Design review of the part built by this model. Coordinates are the model's own, in mm. A direction names the side the tool comes from. Coordinates: 2 decimals unless noted, no trailing zeros. Write each loop counter-clockwise with the first axis right and the second up, starting at its lowest first coordinate (ties: lowest second). Pieces come first, ordered by that corner, then holes. Notation, with made-up numbers: (70, 82) -> (102, 82) arc R21 ccw to (102, 87) -> close; hole circle Ø8 at (78, -27). An arc over 180 degrees is marked (long way). Return JSON: item names as keys, results as strings. Group by question number.
from build123d import *

# Parameters (mm, degrees)
SALIENTE_EXTRUIR1_DEPTH    = 105
SALIENTE_EXTRUIR2_DEPTH    = 5
CROQUIS3_W                 = 140
CROQUIS3_H                 = 105
SALIENTE_EXTRUIR3_DEPTH    = 5
CROQUIS4_W                 = 205
CROQUIS4_H                 = 105
SALIENTE_EXTRUIR5_DEPTH    = 5
CROQUIS5_W                 = 205
CROQUIS5_H                 = 105
SALIENTE_EXTRUIR6_DEPTH    = 5
SALIENTE_EXTRUIR7_DEPTH    = 140
CORTAR_EXTRUIR1_DEPTH      = 273.167228172
CORTAR_EXTRUIR1_DEPTH_BACK = 273.167228172
CROQUIS9_W                 = 20
CROQUIS9_H                 = 17.5
CROQUIS9_W_2               = 50
SALIENTE_EXTRUIR8_DEPTH    = 2.5
CROQUIS10_W                = 20
CROQUIS10_H                = 17.5
CROQUIS10_W_2              = 50
SALIENTE_EXTRUIR9_DEPTH    = 2.5
CORTAR_EXTRUIR2_START      = -5
CORTAR_EXTRUIR2_DEPTH      = 140


with BuildPart() as part:
    # Croquis2 → Saliente-Extruir1 (new body)
    with BuildSketch(Plane(origin=(0, 0, 0), x_dir=(1, 0, 0), z_dir=(0, 1, 0))):
        with BuildLine():
            Line((120, 70), (60, 70))
            add(Edge.make_bspline(
                [(60, 70), (89.76394683, -0.562785514), (120, 50)],
                knots=[0, 0, 0, 1, 1, 1], degree=2))
            Line((120, 50), (200, 50))
            Line((200, 50), (200, 70))
            Line((200, 70), (120, 70))
        make_face()
    extrude(amount=SALIENTE_EXTRUIR1_DEPTH)

    # Croquis2_3 → Saliente-Extruir2 (add)
    with BuildSketch(Plane(origin=(0, 0, 0), x_dir=(1, 0, 0), z_dir=(0, 1, 0))):
        with BuildLine():
            Line((60, 70), (60, -70))
            Line((60, -70), (200, -70))
            Line((200, -70), (200, 50))
            Line((200, 50), (120, 50))
            add(Edge.make_bspline(
                [(60, 70), (89.76394683, -0.562785514), (120, 50)],
                knots=[0, 0, 0, 1, 1, 1], degree=2))
        make_face()
    extrude(amount=SALIENTE_EXTRUIR2_DEPTH)

    # Croquis3 → Saliente-Extruir3 (add)
    with BuildSketch(Plane(origin=(200, 0, 0), x_dir=(0, 0, -1), z_dir=(1, 0, 0))):
        with Locations((0, 52.5)):
            Rectangle(CROQUIS3_W, CROQUIS3_H)
    extrude(amount=SALIENTE_EXTRUIR3_DEPTH)

    # Croquis4 → Saliente-Extruir5 (add)
    with BuildSketch(Plane.XY.offset(70)):
        with Locations((102.5, 52.5)):
            Rectangle(CROQUIS4_W, CROQUIS4_H)
    extrude(amount=SALIENTE_EXTRUIR5_DEPTH)

    # Croquis5 → Saliente-Extruir6 (add)
    with BuildSketch(Plane(origin=(0, 0, -70), x_dir=(-1, 0, 0), z_dir=(0, 0, -1))):
        with Locations((-102.5, 52.5)):
            Rectangle(CROQUIS5_W, CROQUIS5_H)
    extrude(amount=SALIENTE_EXTRUIR6_DEPTH)

    # Croquis6 → Saliente-Extruir7 (add)
    with BuildSketch(Plane.XY.offset(-70)):
        Polygon((60, 5), (0, 75), (0, 70), (60, 0), align=None)
    extrude(amount=SALIENTE_EXTRUIR7_DEPTH)

    # Croquis8 → Cortar-Extruir1 (cut, two sides: drawn at the far end of the back side and taken through both)
    with BuildSketch(Plane.XY.offset(-70).offset(-CORTAR_EXTRUIR1_DEPTH_BACK)):
        Polygon((60, 0), (0, 70), (0, 0), align=None)
    extrude(amount=CORTAR_EXTRUIR1_DEPTH + CORTAR_EXTRUIR1_DEPTH_BACK, mode=Mode.SUBTRACT)

    # Croquis9 → Saliente-Extruir8 (add)
    with BuildSketch(Plane.XY.offset(75)):
        with Locations((10, 87.5)):
            Rectangle(CROQUIS9_W, CROQUIS9_H)
        with Locations((-25, 87.5)):
            Rectangle(CROQUIS9_W_2, CROQUIS9_H)
    extrude(amount=-SALIENTE_EXTRUIR8_DEPTH)

    # Croquis10 → Saliente-Extruir9 (add)
    with BuildSketch(Plane(origin=(0, 0, -75), x_dir=(-1, 0, 0), z_dir=(0, 0, -1))):
        with Locations((-10, 87.5)):
            Rectangle(CROQUIS10_W, CROQUIS10_H)
        with Locations((25, 87.5)):
            Rectangle(CROQUIS10_W_2, CROQUIS10_H)
    extrude(amount=-SALIENTE_EXTRUIR9_DEPTH)

    # Croquis11 → Cortar-Extruir2 (cut)
    with BuildSketch(Plane(origin=(0, 105, 0), x_dir=(1, 0, 0), z_dir=(0, 1, 0)).offset(CORTAR_EXTRUIR2_START)):
        with BuildLine():
            Line((65.571134008, 70), (195, 70))
            Line((195, 70), (195, 55))
            Line((195, 55), (117.1633318, 55))
            add(Edge.make_bspline(
                [(117.1633318, 55), (116.553479191, 53.981059511), (115.34399458, 51.951404655), (113.624065501, 49.181454683), (110.189825419, 44.210450859), (105.056898876, 38.454652942), (100.423455416, 35.264929664), (97.501660631, 34.185491141), (95.327997633, 33.847005409), (93.19350491, 33.972145162), (90.391223635, 34.735002625), (85.948013808, 37.366168652), (78.790008493, 44.736062985), (74.164523658, 52.513426841)],
                knots=[-0.028793704, -0.028793704, -0.028793704, -0.004727786, 0.019338133, 0.06746997, 0.163733644, 0.292085209, 0.388348883, 0.452524666, 0.516700448, 0.580876231, 0.677139905, 0.80549147, 0.998018818, 0.998018818, 0.998018818], degree=2))
            Line((74.164523658, 52.513426841), (65.571134008, 70))
        make_face()
    extrude(amount=-CORTAR_EXTRUIR2_DEPTH, mode=Mode.SUBTRACT)


solid = part.part
Q1. Wall thickness on L1, parallel to Z at x = 110, y = 38; L2, parallel to Z at x = 87.5, y = 38.5; L3, parallel to X at y = 52, z = -50.5: over which ranges is each line inside the solid? List them lowest first.
Q2. For P1, Ø0.8, axis at x = -15.5, z = 73.5, coming from the -Y side; P2, Ø12, axis at x = 80, z = -5.5, coming from the +Y side; P3, Ø4.5, axis at y = 75, z = -62.5, coming from the -X side, all flat-tipped, find the tip position at first contact; note any pin that passes through.
Q3. We need section D-D on y = 54.5. State how many separate pieces and enclosed holes the cut face has, plus the area to 3 significant figures.
Q4. We need section B-B on z = 15.5. Write out the cut boundary in (x, y).
Q5. For faces 1 (the flat face through (157, 51, -55)), 2 (the flat face through (129, 5, 15)), 3 (the flat face through (-25, 88, 72.5)), list the 3-axis set-ups (+Z, -Z, +X, -X, +Y, -Y) from which the entire face can be reached by the end or side of a thin tool; tool diameter is ignored.
Q6. We need section A-A on x = -29.5. Write out the cut boundary in (y, z), plus the area to 3 significant figures.
Q7. We need section C-C on x = 148.5. Write out the cut boundary in (y, z), plus the area to 3 significant figures.
Q8. The part is to be moulded in two halves that separate along Z. For faces 4 (the flat face through (-25, 88, -72.5)), 5 (the flat face through (205, 52, 1)), 6 (the flat face through (108, 53, -75)), 7 (the flat face through (131, 100, -60)), say which applies: +Z half, -Z half, draft (parallel to the pull), parting line (faces both ways), or undercut.
Findings below:
{
 "1": {"L1": "z = -75 to -70, -44.15 to -36.58, 70 to 75", "L2": "z = -75 to -70, -36.49 to -30.7, 70 to 75", "L3": "x = 15.43 to 19.71, 69.55 to 75.39, 114.44 to 205"},
 "2": {"P1": "stops at y = 78.75", "P2": "stops at y = 5", "P3": "stops at x = 0"},
 "3": {"separate pieces": "1", "enclosed holes": "2", "area": "4,130 mm^2"},
 "4": {"outline": "(0, 70) -> (60, 0) -> (205, 0) -> (205, 105) -> (200, 105) -> (200, 5) -> (60, 5) -> (0, 75) -> close"},
 "5": {"face 1": "-Y", "face 2": "+Y", "face 3": "-X, +Y, -Y"},
 "6": {"outline": "(78.75, -75) -> (96.25, -75) -> (96.25, -72.5) -> (78.75, -72.5) -> close; (78.75, 72.5) -> (96.25, 72.5) -> (96.25, 75) -> (78.75, 75) -> close", "area": "87.5 mm^2"},
 "7": {"outline": "(0, -75) -> (105, -75) -> (105, -50) -> (5, -50) -> (5, 70) -> (105, 70) -> (105, 75) -> (0, 75) -> (0, -55) -> (100, -55) -> (100, -70) -> (0, -70) -> close", "area": "2,250 mm^2"},
 "8": {"face 4": "undercut", "face 5": "draft", "face 6": "-Z half", "face 7": "undercut"}
}
